Part model, mm, in its own coordinate system. Face numbers are marked on the shaded views. A direction names the side the tool comes from. Coordinates: 2 decimals unless noted, no trailing zeros. Write each loop counter-clockwise with the first axis right and the second up, starting at its lowest first coordinate (ties: lowest second). Pieces come first, ordered by that corner, then holes. Notation, with made-up numbers: (22, 29) -> (28, 29) arc R25 ccw to (28, 44) -> close; hole circle Ø3 at (12.5, -6). An arc over 180 degrees is marked (long way). Write item = value, one per line.
from build123d import *

# Parameters (mm, degrees)
BOSS_EXTRUDE1_DEPTH = 12
CUT_EXTRUDE1_DEPTH  = 5
CUT_EXTRUDE2_DEPTH  = 5


with BuildPart() as part:
    # Sketch2 → Boss-Extrude1 (new body)
    with BuildSketch(Plane(origin=(0, 0, 0), x_dir=(0, 0, -1), z_dir=(1, 0, 0))):
        Polygon((0, 0), (-15, 0), (-15, 8), (-8, 8), (-8, 10), (0, 10), align=None)
    extrude(amount=BOSS_EXTRUDE1_DEPTH)

    # Sketch3 → Cut-Extrude1 (cut)
    with BuildSketch(Plane(origin=(0, 0, 0), x_dir=(-1, 0, 0), z_dir=(0, 0, -1))):
        Polygon((-3.690598923, 9), (-8.309401077, 9), (-10.618802154, 5), (-8.309401077, 1), (-3.690598923, 1), (-1.381197846, 5), align=None)
    extrude(amount=-CUT_EXTRUDE1_DEPTH, mode=Mode.SUBTRACT)

    # Sketch4 → Cut-Extrude2 (cut)
    with BuildSketch(Plane.XZ):
        Polygon((3.690598923, 6), (8.309401077, 6), (10.618802154, 10), (8.309401077, 14), (3.690598923, 14), (1.381197846, 10), align=None)
    extrude(amount=-CUT_EXTRUDE2_DEPTH, mode=Mode.SUBTRACT)


solid = part.part
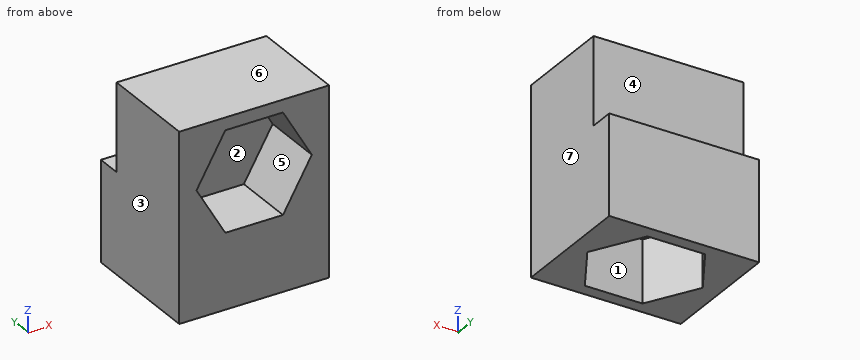
Q1. Mould opens along Z. For the marked faces 5, 6 and 7 say: released by +Z, released by -Z, zero draft, split by the parting line, or undercut.
Model answer:
face_5 = undercut
face_6 = released by +Z
face_7 = zero draft
Q2. Which spindle directions (+Z, -Z, +X, -X, +Y, -Y) get a long thin tool onto all of the face, cutting with end or side? Do the marked faces 1, 2, 3 and 4. Say none if no direction does.
Model answer:
face_1 = -Z
face_2 = -Y
face_3 = +Z, -Z, -X, +Y, -Y
face_4 = +Z, +X, -X, +Y
Q3. Pin check, flat tips, straight feed: pin 1 (2 mm diameter, centred on x = 8.5, z = 11, fed in from +Y); pin 2 (6 mm diameter, centred on x = 6, z = 10, fed in from -Y); pin 3 (2.5 mm diameter, centred on x = 5, y = 3, fed in from -Z). Stop position of each tip, or through.
Model answer:
pin_1 = 8
pin_2 = 5
pin_3 = 5
Q4. Saw through at B-B on x = 7.25. Give the cut face in (y, z).
Model answer:
outline = (0, 0) -> (1, 0) -> (1, 5) -> (9, 5) -> (9, 0) -> (10, 0) -> (10, 8) -> (8, 8) -> (8, 15) -> (0, 15) -> (0, 14) -> (5, 14) -> (5, 6) -> (0, 6) -> close
Q5. Saw through at D-D on z = 7.5. Give the cut face in (x, y).
Model answer:
outline = (0, 0) -> (2.82, 0) -> (2.82, 5) -> (9.18, 5) -> (9.18, 0) -> (12, 0) -> (12, 10) -> (0, 10) -> close
Q6. Saw through at A-A on z = 4.25. Give the cut face in (x, y), and give its area (3 significant figures).
Model answer:
outline = (0, 0) -> (12, 0) -> (12, 10) -> (0, 10) -> close; hole (1.38, 5) -> (3.69, 1) -> (8.31, 1) -> (10.62, 5) -> (8.31, 9) -> (3.69, 9) -> close
area = 64.6 mm²
Q7. Probe line 1 (Y direction, x = 5.25, z = 3); line 2 (Z direction, x = 5, y = 2.25); line 3 (Y direction, x = 10, z = 12). List the from-to ranges inside material, lowest first. Write a range as from..to.
Model answer:
line_1 = 0..1, 9..10
line_2 = 5..6, 14..15
line_3 = 0..8
Q8. Saw through at C-C on y = 1.25. Give the cut face in (x, z).
Model answer:
outline = (0, 0) -> (3.55, 0) -> (3.55, 5) -> (8.45, 5) -> (8.45, 0) -> (12, 0) -> (12, 15) -> (0, 15) -> close; hole (1.38, 10) -> (3.69, 6) -> (8.31, 6) -> (10.62, 10) -> (8.31, 14) -> (3.69, 14) -> close
